from build123d import *

# Parameters (mm, degrees)
F0_W     = 85
F0_H     = 56
F1_DEPTH = 1.6002
F2_R     = 1.397
F3_DEPTH = 25.4
F4_R     = 1.397
F5_DEPTH = 25.4
F6_R     = 2.54


with BuildPart() as f1:
    # F0 (on Top) → F1 (new body)
    with BuildSketch(Plane.XY):
        Rectangle(F0_W, F0_H)
    extrude(amount=F1_DEPTH)

    # F2 (on face) → F3 (cut)
    with BuildSketch(Plane.XY.offset(1.6002)):
        with Locations((-38.9948, 24.5)):
            Circle(F2_R)
        with Locations((-38.9948, -24.4948)):
            Circle(F2_R)
        with Locations((19.0052, 24.4948)):
            Circle(F2_R)
        with Locations((19.0052, -24.4948)):
            Circle(F2_R)
    extrude(amount=-F3_DEPTH, mode=Mode.SUBTRACT)

    # F4 (on face) → F5 (cut)
    with BuildSketch(Plane.XY.offset(1.6002)):
        with Locations((-17, -10)):
            Circle(F4_R)
        with Locations((37.5, 15.5)):
            Circle(F4_R)
    extrude(amount=-F5_DEPTH, mode=Mode.SUBTRACT)

    # F6
    f6_edges = [f1.edges().sort_by_distance(p)[0] for p in [
        (-42.5, -28, 0.8001),
        (42.5, -28, 0.8001),
        (42.5, 28, 0.8001),
        (-42.5, 28, 0.8001),
    ]]
    fillet(f6_edges, radius=F6_R)


solid = f1.part
Work out the finished part from the listing and answer in its coordinate system (mm). Round coordinates to 2 decimals unless told otherwise and drop trailing zeros. Order: outer loops, then holes, each group sorted by start corner. A loop starts at its lowest first (then second) coordinate and runs counter-clockwise, first axis right, second up. Notation, with made-up numbers: M 29,-1 L 40,-1 A19 cw 40,20 Z; hole C -27.75,42 d10. An arc over 180 degrees is marked long. One line per item, written item: value.
Q1. Find section A-A on y = 15.5. Write down the section's boundary in (x, z), then the cut area to 3 significant figures.
Derived:
outline: M -42.5,0 L 36.1,0 L 36.1,1.6 L -42.5,1.6 Z; M 38.9,0 L 42.5,0 L 42.5,1.6 L 38.9,1.6 Z
area: 132 mm²
Q2. Find section B-B on x = 37.5. Write down the section's boundary in (y, z), then the cut area to 3 significant figures.
Derived:
outline: M -28,0 L 14.1,0 L 14.1,1.6 L -28,1.6 Z; M 16.9,0 L 28,0 L 28,1.6 L 16.9,1.6 Z
area: 85.1 mm²
Q3. Determine the mould class of faces 1 (the face through (-1, -28, 1)), 2 (the face through (-1, 28, 1)), 3 (the face through (20.296, -25.03, 0.811)) for opening direction Y: released by +Y, released by -Y, zero draft, split by the parting line, or undercut.
Derived:
face 1: released by -Y
face 2: released by +Y
face 3: undercut
Q4. Straight lines are drawn through the part: line 1 (Y direction, x = 37.5, z = 1.05); line 2 (Y direction, x = -39, z = 0.5). For each, find the intervals that lie inside material, in ascending order.
Derived:
line 1: -28 to 14.1, 16.9 to 28
line 2: -28 to -25.89, -23.1 to 23.1, 25.9 to 28
